Input: dimensioned drawing with shaded views. Units: mm. Origin: part minimum x, y, z. A direction names the side the tool comes from. Coordinates: 2 decimals unless noted, no trailing zeros. Loops run counter-clockwise (first coordinate to the right, second up) from the corner with the lowest first, then second, coordinate; pieces in that order, holes last. Notation, with made-up numbers: (77, 5) - (118, 5) arc R7 cw to (118, 13) - close; hole circle Ø11 at (7.25, 88.25). An arc over 180 degrees is marked (long way). Use one line per item in the form item = value. Start each with the question number.
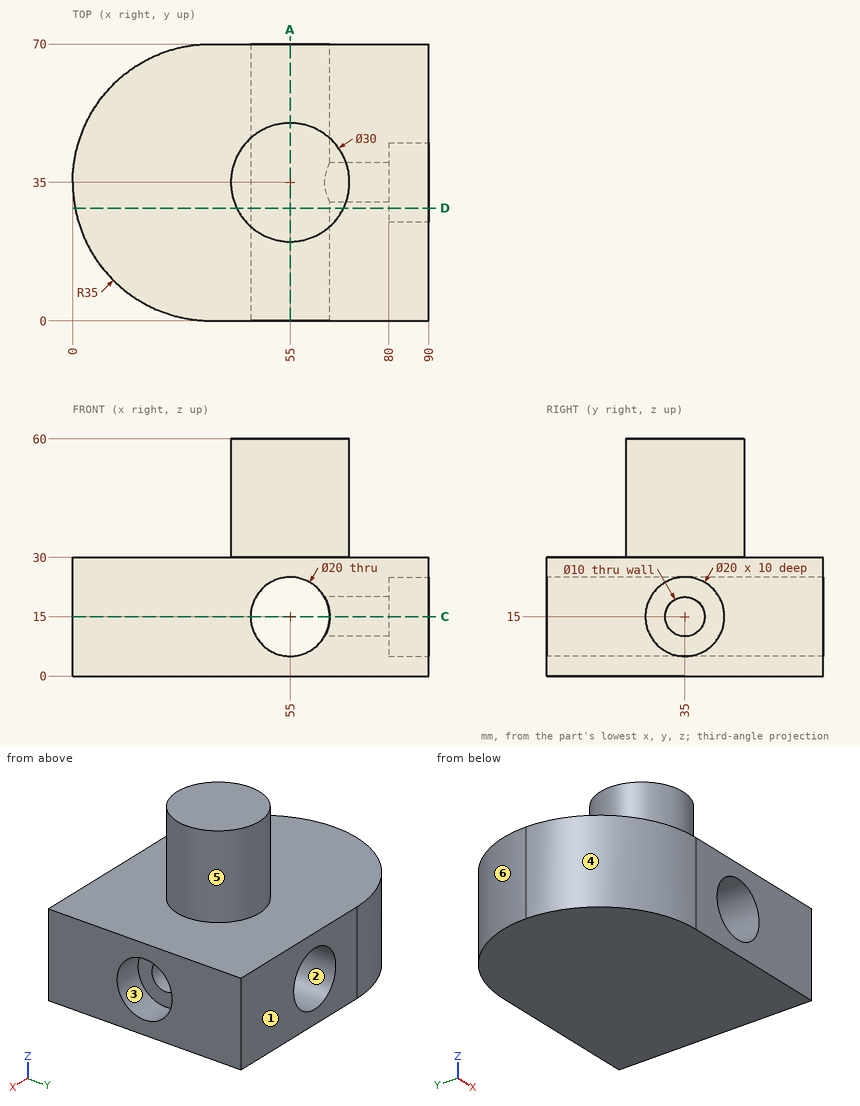
(1) Cut plane D-D, the plane y = 28.5. Output: boundary loops of the cut face in (x, z), plus the area to 3 significant figures.
(2) Cut plane C-C, the plane z = 15. State how many separate pieces and enclosed holes the cut face has, plus the area to 3 significant figures.
(3) Contact query for flat-ended pins moving along their axis: pin 1 (6 mm diameter, centred on y = 39, z = 19.5, fed in from +X); pin 2 (12 mm diameter, centred on x = 61.5, y = 8.5, fed in from +Z); pin 3 (8 mm diameter, centred on x = 59, z = 35, fed in from +Y). Output: stop coordinate, or through.
(4) Mould query, pull axis Y, two halves, no side actions, for the marked faces 1, 2, 3 and 4. Classes: +Y half, -Y half, draft (parallel to the pull), parting line (faces both ways), or undercut.
(5) Access query for the marked faces 5 and 6. Directions: +Z, -Z, +X, -X, +Y, -Y. A direction counts if a zero-diameter tool reaches every point of the face in a straight line with its end or side. Return the directions, or none.
(6) Material intervals for line 1 (Z direction, x = 72, y = 35); line 2 (Z direction, x = 55, y = 34); line 3 (Y direction, x = 72.5, z = 15), sorted ascending.
(7) Cut plane A-A, the plane x = 55. Output: boundary loops of the cut face in (y, z), plus the area to 3 significant figures.
Recorded:
q1.outline = (0.61, 0) - (90, 0) - (90, 7.4) - (80, 7.4) - (80, 22.6) - (90, 22.6) - (90, 30) - (68.52, 30) - (68.52, 60) - (41.48, 60) - (41.48, 30) - (0.61, 30) - close; hole circle Ø20 at (55, 15)
q1.area = 3,030 mm²
q2.separate_pieces = 3
q2.enclosed_holes = 0
q2.area = 4,020 mm²
q3.pin_1 = 80
q3.pin_2 = 30
q3.pin_3 = 50
q4.face_1 = +Y half
q4.face_2 = draft
q4.face_3 = undercut
q4.face_4 = -Y half
q5.face_5 = +Z
q5.face_6 = +Z, -Z, -X, +Y
q6.line_1 = 0 to 10, 20 to 30
q6.line_2 = 0 to 5, 25 to 60
q6.line_3 = 0 to 30, 40 to 70
q7.outline = (0, 0) - (70, 0) - (70, 5) - (0, 5) - close; (0, 25) - (70, 25) - (70, 30) - (50, 30) - (50, 60) - (20, 60) - (20, 30) - (0, 30) - close
q7.area = 1,600 mm²
